```python
from build123d import *

# Parameters (mm, degrees)
SKETCH_R  = 9.875
PAD_DEPTH = 1


with BuildPart() as part:
    # Sketch → Pad (new body, symmetric)
    with BuildSketch(Plane.XZ):
        with BuildLine():
            Line((-15, -12), (1.5, -12))
            Line((1.5, 12), (1.5, -12))
            Line((1.5, 12), (-15, 12))
            ThreePointArc((-15, 12), (-27, 0), (-15, -12))
        make_face()
        with Locations((-15, 0)):
            Circle(SKETCH_R, mode=Mode.SUBTRACT)
    extrude(amount=PAD_DEPTH, both=True)


solid = part.part
```
For this review, take the finished solid that the model builds, in its own axes (mm). Round coordinates to 2 decimals unless told otherwise and drop trailing zeros. Order: outer loops, then holes, each group sorted by start corner. A loop starts at its lowest first (then second) coordinate and runs counter-clockwise, first axis right, second up. Notation, with made-up numbers: (49.25, 13.5) -> (103.25, 13.5) arc R25 cw to (103.25, 25.5) -> close; hole circle Ø2 at (-7.75, -35). An arc over 180 degrees is marked (long way). Use a Markdown table: item, result.
Item 1: Draft analysis for pull direction Z (two halves, no side actions). For faces 1 (the flat face through (-7, 0, -12)), 2 (the flat face through (-7, 0, 12)), 3 (the cylindrical face through (-5.581, 0.014, 2.966)), 4 (the flat face through (1.5, 0, 0)), state which applies: +Z half, -Z half, draft (parallel to the pull), parting line (faces both ways), or undercut.
Resolved:
| item | result |
|---|---|
| face 1 | -Z half |
| face 2 | +Z half |
| face 3 | undercut |
| face 4 | draft |
Item 2: For line 1 along Z through (x, y) = (-15, 0.15) (3 decimals); line 2 along Z through (x, y) = (-7, -0.2); line 3 along X through (y, z) = (0.5, 0.5), list the stretches that pass through material, from the lowest coordinate up. Write a range as [from, to].
Resolved:
| item | result |
|---|---|
| line 1 | z = [-12, -9.875], [9.875, 12] |
| line 2 | z = [-12, -5.79], [5.79, 12] |
| line 3 | x = [-26.99, -24.86], [-5.14, 1.5] |
Item 3: Take a section at B-B (x = -21). State the section outline as (y, z) points.
Resolved:
| item | result |
|---|---|
| outline | (-1, -10.39) -> (1, -10.39) -> (1, -7.84) -> (-1, -7.84) -> close; (-1, 7.84) -> (1, 7.84) -> (1, 10.39) -> (-1, 10.39) -> close |
Item 4: Take a section at A-A (z = 0). State the section outline as (x, y) points (3 decimals), plus the area to 3 significant figures.
Resolved:
| item | result |
|---|---|
| outline | (-27, -1) -> (-24.875, -1) -> (-24.875, 1) -> (-27, 1) -> close; (-5.125, -1) -> (1.5, -1) -> (1.5, 1) -> (-5.125, 1) -> close |
| area | 17.5 mm² |
